Read the model definition and answer for the solid it produces. Units are mm, in the model's axes. A direction names the side the tool comes from. Coordinates: 2 decimals unless noted, no trailing zeros. Write each loop counter-clockwise with the first axis right and the second up, starting at its lowest first coordinate (ties: lowest second). Pieces come first, ordered by that corner, then holes.
1) Each of these flat-tipped pins is pushed along its axis until it touches: pin 1 Ø6.5 at (x, y) = (-59.07, -28.76) entering from -Z; pin 2 Ø6.5 at (x, y) = (-11.93, -75.9) entering from +Z. Where does it stop, or does it pass through?
2) The part is cut by section C-C (y = -46.5). Determine the outline of the cut face in (x, z), then the cut area to 3 significant figures.
3) Which of the six approach directions +Z, -Z, +X, -X, +Y, -Y give full straight-line access (tool end or side, diameter ignored) to faces 4 (the face through (-73, -49, 5)), 5 (the face through (-63.2, -24.54, 3.31))?
4) The part is cut by section B-B (z = 5). Determine the outline of the cut face in (x, y).
5) Determine the mould class of faces 1 (the face through (-71.496, -11.253, 4.827)), 2 (the face through (-14, -49, 9.52)), 3 (the face through (-53.975, -59.988, 7.999)) for opening direction X: +X half, -X half, draft (parallel to the pull), parting line (faces both ways), or undercut.
6) The part is cut by section A-A (x = -35.5). Determine the outline of the cut face in (y, z).
7) Find the intervals of material crossed by line 1 (Y direction, x = -59.07, z = 7.95); line 2 (X direction, y = -45, z = 3.25); line 3 (Y direction, x = -35, z = 2.5), in increasing order.
Autodesk Inventor part; units mm, degrees
ref_plane "YZ Plane" through (0, 0, 0) normal (1, 0, 0) x (0, 1, 0)
ref_plane "XZ Plane" through (0, 0, 0) normal (0, 1, 0) x (-1, 0, 0)
ref_plane "XY Plane" through (0, 0, 0) normal (0, 0, 1) x (1, 0, 0)
sketch "Esboço1" plane through (0, 0, 0) normal (0, 0, 1) x (1, 0, 0)
  line L0 (-33, -50) -> (-33, 950)
  line L1 (47, -50) -> (47, 950)
  line L2 (-73, -89.8276) -> (47, -89.8276)
  line L3 (47, -9.8276) -> (-73, -9.8276)
  line L4 (-73, -9.8276) -> (-73, -89.8276)
  line L5 (47, -89.8276) -> (47, -9.8276)
  point P0 (0, 0)
  dimension "d0" = 120
  dimension "d1" = 120
  dimension "d2" = 80
extrude "Extrusão1" add sketch "Esboço1" along normal blind 9.52
sketch "Esboço9" plane through (0, 0, 0) normal (0, 0, -1) x (-1, 0, 0)
  line L0 (65, -22.8276) -> (6, -22.8276)
  line L1 (6, -22.8276) -> (6, -81.8276)
  line L2 (6, -81.8276) -> (65, -81.8276)
  line L3 (65, -81.8276) -> (65, -22.8276)
  line L4 (65, -22.8276) -> (6, -81.8276) construction
  line L5 (6, -22.8276) -> (65, -81.8276) construction
  line L6 (65, -52.3276) -> (6, -52.3276) construction
  line L7 (35.5, -22.8276) -> (35.5, -81.8276) construction
  circle A0 centre (59.07, -28.7576) radius 2.5
  circle A1 centre (59.07, -75.8976) radius 2.5
  circle A2 centre (11.93, -28.7576) radius 2.5
  circle A3 centre (11.93, -75.8976) radius 2.5
  line L8 (73, -9.8276) -> (73, -89.8276)
  line L9 (73, -89.8276) -> (-47, -89.8276)
  circle A4 centre (35.5, -52.3276) radius 20
  point P0 (0, 0)
  dimension "d72" = 59
  dimension "d73" = 59
  dimension "d74" = 5
  dimension "d75" = 5
  dimension "d76" = 5
  dimension "d77" = 5
  dimension "d78" = 23.57
  dimension "d79" = 23.57
  dimension "d80" = 23.57
  dimension "d81" = 23.57
  dimension "d82" = 23.57
  dimension "d83" = 23.57
  dimension "d84" = 23.57
  dimension "d85" = 23.57
  dimension "d86" = 8
  dimension "d87" = 8
  dimension "d88" = 40
extrude "Extrusão6" cut sketch "Esboço9" against normal blind 6.52
sketch "Esboço10" plane through (-35.5, -52.3276, 0) normal (0, 0, -1) x (-1, 0, 0)
  circle A0 centre (0, 0) radius 20
  circle A1 centre (0, 0) radius 20
  circle A2 centre (23.57, -23.57) radius 2.5
  circle A3 centre (23.57, -23.57) radius 2.5
  circle A4 centre (23.57, 23.57) radius 2.5
  circle A5 centre (23.57, 23.57) radius 2.5
  circle A6 centre (-23.57, 23.57) radius 2.5
  circle A7 centre (-23.57, 23.57) radius 2.5
  circle A8 centre (-23.57, -23.57) radius 2.5
  circle A9 centre (-23.57, -23.57) radius 2.5
  point P0 (-35.5, 52.3276)
extrude "Extrusão7" cut sketch "Esboço10" against normal through all
fillet "Arredondamento1" radius 6 4 edges at (-65, -22.8276, 3.26) (-65, -81.8276, 3.26) (-6, -22.8276, 3.26) (-6, -81.8276, 3.26)
fillet "Arredondamento2" radius 5 2 edges at (-73, -9.8276, 4.76) (-73, -89.8276, 4.76)
equation "\"d0\" = d1"
equation "\"d79\" = d78"
equation "\"d80\" = d78"
equation "\"d81\" = d78"
equation "\"d82\" = d78"
equation "\"d83\" = d78"
equation "\"d84\" = d78"
equation "\"d85\" = d78"
properties part number "SUPORTE_MOTOR_EIXO_Y_1"
Reported:
1. pin 1: stops at z = 6.52
1. pin 2: stops at z = 9.52
2. outline: (-73, 0) - (-65, 0) - (-65, 6.52) - (-54.63, 6.52) - (-54.63, 9.52) - (-73, 9.52) - close; (-16.37, 6.52) - (-6, 6.52) - (-6, 0) - (47, 0) - (47, 9.52) - (-16.37, 9.52) - close
2. area: 643 mm2
3. face 4: +Z, -Z, -X, +Y, -Y
3. face 5: -Z
4. outline: (-73, -84.83) arc R5 ccw to (-68, -89.83) - (47, -89.83) - (47, -9.83) - (-68, -9.83) arc R5 ccw to (-73, -14.83) - close; hole (-65, -75.83) arc R6 ccw to (-59, -81.83) - (-12, -81.83) arc R6 ccw to (-6, -75.83) - (-6, -28.83) arc R6 ccw to (-12, -22.83) - (-59, -22.83) arc R6 ccw to (-65, -28.83) - close
5. face 1: -X half
5. face 2: draft
5. face 3: undercut
6. outline: (-89.83, 0) - (-81.83, 0) - (-81.83, 6.52) - (-72.33, 6.52) - (-72.33, 9.52) - (-89.83, 9.52) - close; (-32.33, 6.52) - (-22.83, 6.52) - (-22.83, 0) - (-9.83, 0) - (-9.83, 9.52) - (-32.33, 9.52) - close
7. line 1: y = -89.83 to -78.4, -73.4 to -31.26, -26.26 to -9.83
7. line 2: x = -73 to -65, -6 to 47
7. line 3: y = -89.83 to -81.83, -22.83 to -9.83
